Check sheet for the modelled part. Datum: model origin and axes. Units: mm. A direction names the side the tool comes from. Give positions to 0.01 mm unless a question says otherwise; leave off trailing zeros. Write each loop counter-clockwise with the first axis right and the second up, starting at its lowest first coordinate (ties: lowest second). Pieces come first, ordered by that corner, then holes. Notation, with made-up numbers: (87, 67.25) -> (124, 67.25) arc R18 ccw to (124, 82.25) -> close; hole circle Ø2 at (55.25, 15.25). An arc over 180 degrees is marked (long way). Return JSON: item names as keys, results as strings.
Autodesk Inventor part; units mm, degrees
ref_plane "YZ Plane" through (0, 0, 0) normal (1, 0, 0) x (0, 1, 0)
ref_plane "XZ Plane" through (0, 0, 0) normal (0, 1, 0) x (-1, 0, 0)
ref_plane "XY Plane" through (0, 0, 0) normal (0, 0, 1) x (1, 0, 0)
sketch "Sketch1" plane through (0, 0, 0) normal (0, 0, 1) x (1, 0, 0)
  line L0 (0, 0) -> (0, 9)
  line L1 (0, 9) -> (-2.7, 9)
  line L2 (-2.7, 9) -> (-2.7, 6)
  line L3 (-2.7, 6) -> (-1.5, 6)
  line L4 (-1.5, 6) -> (-1.5, 0)
  line L5 (-1.5, 0) -> (0, 0)
  dimension "d0" = 6
  dimension "d1" = 3
  dimension "d2" = 1.5
  dimension "d3" = 2.7
revolve "Revolution1" add sketch "Sketch1" angle 360 about axis through (0, 0, 0) along (0, 1, 0)
sketch "Sketch2" plane through (0, 9, 0) normal (0, 1, 0) x (1, 0, 0)
  line L0 (-0.7217, -1.25) -> (-1.4434, 0)
  line L1 (-1.4434, 0) -> (-0.7217, 1.25)
  line L2 (-0.7217, 1.25) -> (0.7217, 1.25)
  line L3 (0.7217, 1.25) -> (1.4434, 0)
  line L4 (1.4434, 0) -> (0.7217, -1.25)
  line L5 (0.7217, -1.25) -> (-0.7217, -1.25)
  point P0 (0, 0)
  point P1 (0, 0)
  dimension "d5" = 2.5
extrude "Extrusion1" cut sketch "Sketch2" against normal blind 2
fillet "Fillet1" radius 0.3 6 edges at (0, 9, -1.25) (1.0825, 9, -0.625) (1.0825, 9, 0.625) (0, 9, 1.25) (-1.0825, 9, 0.625) (-1.0825, 9, -0.625)
fillet "Fillet2" radius 0.3 1 edges at (2.7, 9, 0)
thread "Thread1"
properties part number "Screw_M3X6_SS_HEX" material "Stainless Steel"
(1) Depth check by flat-ended pin: pin 1 Ø1 at (x, y) = (1.5, 2.5) entering from +Z; pin 2 Ø3 at (x, z) = (2, 1.5) entering from -Y; pin 3 Ø0.7 at (x, y) = (-0.5, 8) entering from +Z; pin 4 Ø3 at (x, y) = (-2, 6.5) entering from -Z. Enter the tip coordinate at first touch or a pass-through.
Reply:
{"pin 1": "z = 1.12", "pin 2": "y = 0", "pin 3": "z = 2.7", "pin 4": "z = -2.65"}
(2) Thickness scan on L1, parallel to Y at x = 1.2, z = 0.2; L2, parallel to Y at x = -0.85, z = -1.9; L3, parallel to X at y = 8.75, z = 0.35. Record the ranges inside material, lowest first.
Reply:
{"L1": "0 to 7", "L2": "6 to 9", "L3": "-2.67 to -1.25, 1.25 to 2.67"}
(3) Release check for a two-part mould opening along Z. For faces 1 (the flat face through (0, 9, -2)), 2 (the cylindrical face through (0.585, 7.331, 2.636)), 3 (the flat face through (-1.088, 7.862, -0.616)) record: pulls with the +Z half, pulls with the -Z half, needs draft (parallel to the pull), parting line crosses it, or undercut.
Reply:
{"face 1": "needs draft", "face 2": "parting line crosses it", "face 3": "undercut"}
(4) Cross-section at A-A on x = 0. Enter the section's corners in (y, z).
Reply:
{"outline": "(0, -1.5) -> (6, -1.5) -> (6, -2.7) -> (8.7, -2.7) arc R0.3 ccw to (9, -2.4) -> (9, -1.55) arc R0.3 ccw to (8.7, -1.25) -> (7, -1.25) -> (7, 1.25) -> (8.7, 1.25) arc R0.3 ccw to (9, 1.55) -> (9, 2.4) arc R0.3 ccw to (8.7, 2.7) -> (6, 2.7) -> (6, 1.5) -> (0, 1.5) -> close"}
(5) Cross-section at B-B on y = 3.25. Enter the section's corners in (x, z), then the cut area to 3 significant figures.
Reply:
{"outline": "circle Ø3 at (0, 0)", "area": "7.07 mm^2"}
(6) Set-up check for faces 4 (the flat face through (0, 0, 0)), 5 (the flat face through (-1.08, 7.86, 0.63)), 6 (the flat face through (-1.2, 6, -1.2)): record each of +Z, -Z, +X, -X, +Y, -Y from which the full face is reachable in a straight line by a thin tool's end or side.
Reply:
{"face 4": "+Z, -Z, +X, -X, -Y", "face 5": "+Y", "face 6": "-Y"}
